from build123d import *

# Parameters (mm, degrees)
BOSS_EXTRUDE1_DEPTH         = 25
CUT_EXTRUDE1_DEPTH          = 21
CUT_EXTRUDE2_DEPTH          = 16.25
M3_TAPPED_HOLE1_D           = 2.5
M3_TAPPED_HOLE1_DEPTH       = 8.5
M3_TAPPED_HOLE1_CSINK_D     = 3.05
M3_TAPPED_HOLE1_CSINK_ANGLE = 90
M3_TAPPED_HOLE1_TIP         = 0.751075774
SKETCH5_R                   = 7
BOSS_EXTRUDE2_DEPTH         = 5
SKETCH6_R                   = 4.5
CUT_EXTRUDE3_DEPTH          = 7
SKETCH7_R                   = 2.15
CUT_EXTRUDE4_DEPTH          = 4.5
CHAMFER2_SIZE               = 1.5
CHAMFER2_SIZE2              = 3
CUT_EXTRUDE5_REACH          = 64.204
CUT_EXTRUDE5_END_RADIUS     = 3.5
SKETCH8_R                   = 0.9
CHAMFER2_OF_MIRROR1_SIZE2   = 1.5
CHAMFER2_OF_MIRROR1_SIZE    = 3
CHAMFER3_SIZE               = 4.5
CHAMFER3_SIZE2              = 3
CHAMFER4_SIZE               = 0.75


with BuildPart() as part:
    # Sketch1 → Boss-Extrude1 (new body)
    with BuildSketch(Plane.XY):
        with BuildLine():
            Line((-36.885, 15), (8.115, 15))
            ThreePointArc((8.115, 15), (23.115, 0), (8.115, -15))
            Line((8.115, -15), (-36.885, -15))
            ThreePointArc((-36.885, -15), (-51.885, 0), (-36.885, 15))
        make_face()
    extrude(amount=BOSS_EXTRUDE1_DEPTH)

    # Sketch2 → Cut-Extrude1 (cut)
    with BuildSketch(Plane.XY.offset(25)):
        with BuildLine():
            Line((-3.5, 11.5), (-38.5, 11.5))
            Line((-38.5, 11.5), (-38.5, 4.9))
            Line((-38.5, 4.9), (-45.3, 4.9))
            Line((-45.3, 4.9), (-45.3, -4.9))
            Line((-45.3, -4.9), (-38.5, -4.9))
            Line((-38.5, -4.9), (-38.5, -11.5))
            Line((-38.5, -11.5), (-33.385, -11.5))
            Line((-33.385, -11.5), (-33.385, -16.5))
            Line((-33.385, -16.5), (-14.635, -16.5))
            Line((-14.635, -16.5), (-14.635, -11.5))
            Line((-14.635, -11.5), (-3.5, -11.5))
            Line((-3.5, -11.5), (-3.5, -10.175))
            ThreePointArc((-3.5, -10.175), (-3.031207817, -8.425205963), (-1.750411903, -7.144148936))
            ThreePointArc((-1.750411903, -7.144148936), (2.373617184, 0), (-1.750411903, 7.144148936))
            ThreePointArc((-1.750411903, 7.144148936), (-3.031207817, 8.425205963), (-3.5, 10.175))
            Line((-3.5, 10.175), (-3.5, 11.5))
        make_face()
    extrude(amount=-CUT_EXTRUDE1_DEPTH, mode=Mode.SUBTRACT)

    # Sketch2<3> → Cut-Extrude2 (cut)
    with BuildSketch(Plane.XY.offset(25)):
        with BuildLine():
            ThreePointArc((3.474243454, 9.75116935), (1.562702039, 7.043233352), (-1.750411903, 7.144148936))
            ThreePointArc((-1.750411903, 7.144148936), (2.373617184, 0), (-1.750411903, -7.144148936))
            ThreePointArc((-1.750411903, -7.144148936), (1.562702039, -7.043233352), (3.474243454, -9.75116935))
            ThreePointArc((3.474243454, -9.75116935), (4.469872156, -11.798465751), (6.514146928, -12.800283959))
            ThreePointArc((6.514146928, -12.800283959), (9.174878964, -12.856385829), (11.79050107, -12.365301933))
            Line((11.79050107, -12.365301933), (11.391974761, -11.675088283))
            ThreePointArc((11.391974761, -11.675088283), (12.489911717, -7.576974761), (16.588025239, -8.674911717))
            Line((16.588025239, -8.674911717), (16.986551548, -9.365125367))
            ThreePointArc((16.986551548, -9.365125367), (21.015, 0), (16.986551548, 9.365125367))
            Line((16.986551548, 9.365125367), (16.588025239, 8.674911717))
            ThreePointArc((16.588025239, 8.674911717), (12.489911717, 7.576974761), (11.391974761, 11.675088283))
            Line((11.391974761, 11.675088283), (11.79050107, 12.365301933))
            ThreePointArc((11.79050107, 12.365301933), (9.174878964, 12.856385829), (6.514146928, 12.800283959))
            ThreePointArc((6.514146928, 12.800283959), (4.469872156, 11.798465751), (3.474243454, 9.75116935))
        make_face()
    extrude(amount=-CUT_EXTRUDE2_DEPTH, mode=Mode.SUBTRACT)

    # M3 Tapped Hole1
    with Locations(Plane.XY.offset(25)):
        with Locations((-42.76, 10.175), (-42.76, -10.175), (0, -10.175), (0, 10.175), (13.99, 10.175), (13.99, -10.175)):
            CounterSinkHole(M3_TAPPED_HOLE1_D / 2, M3_TAPPED_HOLE1_CSINK_D / 2, depth=M3_TAPPED_HOLE1_DEPTH, counter_sink_angle=M3_TAPPED_HOLE1_CSINK_ANGLE)
            with Locations((0, 0, -(M3_TAPPED_HOLE1_DEPTH + M3_TAPPED_HOLE1_TIP / 2))):  # 118° drill point
                Cone(0, M3_TAPPED_HOLE1_D / 2, M3_TAPPED_HOLE1_TIP, mode=Mode.SUBTRACT)

    # Sketch5 → Boss-Extrude2 (add)
    with BuildSketch(Plane(origin=(0, 15, 0), x_dir=(1, 0, 0), z_dir=(0, 1, 0))):
        with Locations((0, -12.5)):
            Circle(SKETCH5_R)
    boss_extrude2 = extrude(amount=BOSS_EXTRUDE2_DEPTH)

    # Sketch6 → Cut-Extrude3 (cut)
    with BuildSketch(Plane(origin=(0, 20, 0), x_dir=(1, 0, 0), z_dir=(0, 1, 0))):
        with Locations(Location((0, -12.5, 0), (0, 0, 180))):
            Circle(SKETCH6_R)
    cut_extrude3 = extrude(amount=-CUT_EXTRUDE3_DEPTH, mode=Mode.SUBTRACT)

    # Sketch7 → Cut-Extrude4 (cut)
    with BuildSketch(Plane(origin=(0, 13, 0), x_dir=(1, 0, 0), z_dir=(0, 1, 0))):
        with Locations(Location((0, -12.5, 0), (0, 0, 180))):
            Circle(SKETCH7_R)
    cut_extrude4 = extrude(amount=-CUT_EXTRUDE4_DEPTH, mode=Mode.SUBTRACT)

    # Chamfer2
    chamfer2_edges = [part.edges().sort_by_distance(p)[0] for p in [
        (2.15, 13, 12.5),
    ]]
    chamfer2_side = [part.faces().sort_by_distance(p)[0] for p in [
        (4.372720779, 13, 12.5),
    ]]
    chamfer(chamfer2_edges, length=CHAMFER2_SIZE, length2=CHAMFER2_SIZE2, reference=chamfer2_side[0])

    # Cut-Extrude5: up to this cylinder (the profile starts inside it)
    cut_extrude5_end = Plane(origin=(0, 10.175, 12.5), z_dir=(0, 0, 1)) * Cylinder(CUT_EXTRUDE5_END_RADIUS, 136.408, mode=Mode.PRIVATE)
    # Sketch8 → Cut-Extrude5 (cut, up to the surface)
    with BuildSketch(Plane(origin=(0, 8.5, 0), x_dir=(1, 0, 0), z_dir=(0, 1, 0)), mode=Mode.PRIVATE) as cut_extrude5_sk1:
        with Locations(Location((0, -12.5, 0), (0, 0, 180))):
            Circle(SKETCH8_R)
    cut_extrude5_tool1 = extrude(cut_extrude5_sk1.sketch, amount=-CUT_EXTRUDE5_REACH, mode=Mode.PRIVATE) & cut_extrude5_end
    cut_extrude5 = cut_extrude5_tool1.solids().sort_by_distance((0, 8.5, 12.5))[0]
    add(cut_extrude5, mode=Mode.SUBTRACT)

    # Mirror1: Boss-Extrude2, Cut-Extrude3, Cut-Extrude4, Cut-Extrude5 across plane
    add(boss_extrude2.mirror(Plane.ZX))
    add(cut_extrude3.mirror(Plane.ZX), mode=Mode.SUBTRACT)
    add(cut_extrude4.mirror(Plane.ZX), mode=Mode.SUBTRACT)
    add(cut_extrude5.mirror(Plane.ZX), mode=Mode.SUBTRACT)

    # Chamfer2 of Mirror1
    chamfer2_of_mirror1_edges = [part.edges().sort_by_distance(p)[0] for p in [
        (2.15, -13, 12.5),
    ]]
    chamfer(chamfer2_of_mirror1_edges, length=CHAMFER2_OF_MIRROR1_SIZE, length2=CHAMFER2_OF_MIRROR1_SIZE2)

    # Chamfer3
    chamfer3_edges = [part.edges().sort_by_distance(p)[0] for p in [
        (-14.385, 15, 0),
        (23.115, 0, 0),
        (-14.385, -15, 0),
        (-51.885, 0, 0),
    ]]
    chamfer3_side = [part.faces().sort_by_distance(p)[0] for p in [
        (-14.385, 0, 0),
    ]]
    chamfer(chamfer3_edges, length=CHAMFER3_SIZE, length2=CHAMFER3_SIZE2, reference=chamfer3_side[0])

    # Chamfer4
    chamfer4_edges = [part.edges().sort_by_distance(p)[0] for p in [
        (-7, 15, 12.5),
        (-7, 20, 12.5),
        (-7, -20, 12.5),
        (-7, -15, 12.5),
    ]]
    chamfer(chamfer4_edges, length=CHAMFER4_SIZE)


solid = part.part
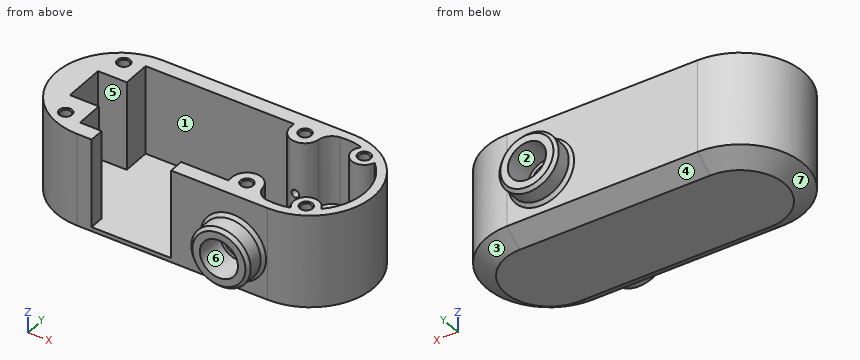
Input: part model. Units: mm. Frame: model coordinates. Face numbers are marked on the shaded views. A direction names the side the tool comes from. Give positions to 0.01 mm unless a question says otherwise; leave off trailing zeros. Order: outer loops, then holes, each group sorted by start corner. A loop starts at its lowest first (then second) coordinate and runs counter-clockwise, first axis right, second up.
Q1. Section B-B on x = -21. Output: boundary loops of the cut face in (y, z).
Checked values:
outline: (-15, 3) - (-10.5, 0) - (10.5, 0) - (15, 3) - (15, 25) - (11.5, 25) - (11.5, 4) - (-15, 4) - close
Q2. Ray query, probe 1 along Y at (x, z) = (13.99, 19.5) (3 decimals); probe 2 along Y at (x, z) = (-34, 5.5); probe 3 along X at (y, z) = (-10, 22). Return the intervals inside material, ascending.
Checked values:
probe 1: y = -13.802 to -11.425, -8.925 to -7.175, 7.175 to 8.925, 11.425 to 13.802
probe 2: y = -15 to -11.5, 11.5 to 15
probe 3: x = -48.07 to -44, -41.52 to -38.5, -3.5 to -1.24, 1.24 to 3.51, 11 to 12.75, 15.23 to 19.3
Q3. Section A-A on y = 0. Output: boundary loops of the cut face in (x, z) (3 decimals), and give its area (3 significant figures).
Checked values:
outline: (-51.885, 3) - (-47.385, 0) - (18.615, 0) - (23.115, 3) - (23.115, 25) - (21.015, 25) - (21.015, 8.75) - (2.374, 8.75) - (2.374, 4) - (-45.3, 4) - (-45.3, 25) - (-51.885, 25) - close
area: 557 mm2
Q4. Draft query along X for the marked faces 1, 2, 3 and 4. Return one class per face: +X half, -X half, draft (parallel to the pull), parting line (faces both ways), or undercut.
Checked values:
face 1: undercut
face 2: undercut
face 3: +X half
face 4: draft
Q5. Contact query for flat-ended pins moving along their axis: pin 1 Ø5 at (y, z) = (1.5, 18) entering from +X (3 decimals); pin 2 Ø3.5 at (x, z) = (0.5, 13) entering from +Y; pin 3 Ø1.5 at (x, z) = (-21.5, 3) entering from +Y; pin 4 Ø4.5 at (x, z) = (-0.5, 13.5) entering from -Y. Output: stop coordinate, or through.
Checked values:
pin 1: stops at x = 23.115
pin 2: stops at y = 10.61
pin 3: stops at y = 15
pin 4: stops at y = -12.44
Q6. Set-up query: the marked faces 5, 6 and 7. Return all of +Z, -Z, +X, -X, +Y, -Y with unobstructed straight access to the full face (end or side cutting, diameter ignored); none if empty.
Checked values:
face 5: +Z
face 6: -Y
face 7: -Z, -X
Q7. Section D-D on z = 12.5. State how many separate pieces and enclosed holes the cut face has, and give its area (3 significant figures).
Checked values:
separate pieces: 3
enclosed holes: 0
area: 641 mm2
Q8. Section C-C on z = 2.25. Output: boundary loops of the cut face in (x, y) (3 decimals).
Checked values:
outline: (-36.885, -13.875) - (8.115, -13.875) arc R13.875 ccw to (8.115, 13.875) - (-36.885, 13.875) arc R13.875 ccw to start
